Answer from the drawing. Dimensions are ordinates in mm from the lowest x, y and z of the part. A direction names the side the tool comes from. Coordinates: 2 decimals unless noted, no trailing zeros. Loops run counter-clockwise (first coordinate to the right, second up) from the corner with the lowest first, then second, coordinate; pieces in that order, holes last. Notation, with made-up numbers: (43, 45.5) - (80, 45.5) arc R37 cw to (80, 82.5) - close; hole circle Ø1 at (-28, -0.5). An arc over 180 degrees is marked (long way). Use one line per item in the form item = value. Start each with the question number.
1) A cutting plane is placed at C-C (y = 38.5). Give the vertices of the cut face in (x, z) (1 decimal).
2) A cutting plane is placed at A-A (y = 18.5). Give the vertices of the cut face in (x, z) (1 decimal), and give its area (3 significant figures).
3) A cutting plane is placed at D-D (x = 66.5). Give the vertices of the cut face in (y, z), and give its area (4 significant figures).
4) Consider line 1 (Z direction, x = 75, y = 74); line 2 (X direction, y = 22.5, z = 17); line 3 (Z direction, x = 79.5, y = 32.5). Determine where each line is inside the solid, lowest interval first.
5) Which of the six approach directions +Z, -Z, +X, -X, +Y, -Y give full straight-line access (tool end or side, diameter ignored) to the marked faces 1, 2 and 3?
6) Each of these flat-tipped pins is pushed along its axis until it touches: P1, Ø1, axis at y = 50.5, z = 19.5, coming from the -X side; P2, Ø10, axis at x = 41, z = 48, coming from the -Y side; P3, Ø7.5, axis at x = 70.5, z = 7.5, coming from the -Y side. Where does it stop, or does it pass through?
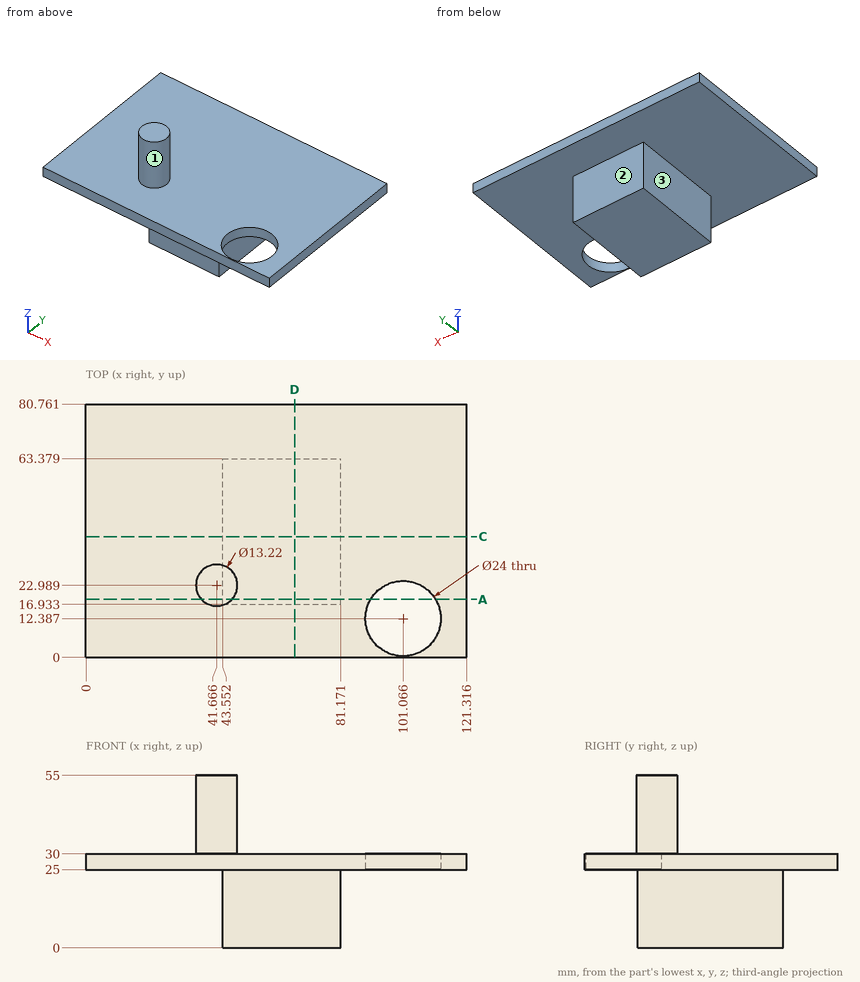
Found:
q1.outline = (0, 25) - (43.6, 25) - (43.6, 0) - (81.2, 0) - (81.2, 25) - (121.3, 25) - (121.3, 30) - (0, 30) - close
q2.outline = (0, 25) - (43.6, 25) - (43.6, 0) - (81.2, 0) - (81.2, 25) - (90.7, 25) - (90.7, 30) - (46.5, 30) - (46.5, 55) - (36.8, 55) - (36.8, 30) - (0, 30) - close; (111.4, 25) - (121.3, 25) - (121.3, 30) - (111.4, 30) - close
q2.area = 1,690 mm^2
q3.outline = (0, 25) - (16.93, 25) - (16.93, 0) - (63.38, 0) - (63.38, 25) - (80.76, 25) - (80.76, 30) - (0, 30) - close
q3.area = 1,565 mm^2
q4.line_1 = 25 to 30
q4.line_2 = 43.55 to 81.17
q4.line_3 = 0 to 30
q5.face_1 = +Z
q5.face_2 = -Z, +X, -X, +Y
q5.face_3 = -Z, -X, +Y, -Y
q6.P1 = 43.55
q6.P2 = 16.38
q6.P3 = 16.93
